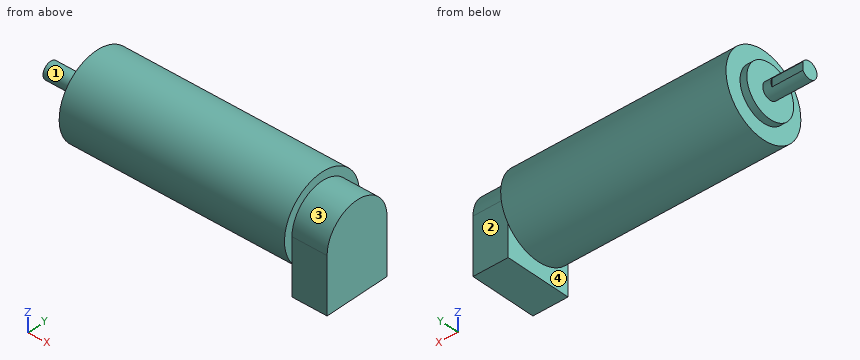
from build123d import *

# Parameters (mm, degrees)
SKETCH_2_R          = 20
EXTRUDE_1_DEPTH     = 109
EXTRUDE_2_DEPTH     = 17
SKETCH_5_R          = 12.5
EXTRUDE_3_DEPTH     = 3.3
SKETCH_6_R          = 4
EXTRUDE_4_DEPTH     = 19
CUT_EXTRUDE_START   = -15
CUT_EXTRUDE_1_DEPTH = 15


with BuildPart() as part:
    # 草图2 → 凸台-拉伸1 (new body)
    with BuildSketch(Plane(origin=(0, 0, 0), x_dir=(0, 0, -1), z_dir=(1, 0, 0))):
        Circle(SKETCH_2_R)
    extrude(amount=EXTRUDE_1_DEPTH)

    # 草图4 → 凸台-拉伸2 (add)
    with BuildSketch(Plane(origin=(109, 0, 0), x_dir=(0, 0, -1), z_dir=(1, 0, 0))):
        with BuildLine():
            Line((0, 16), (27, 16))
            Line((27, 16), (27, -16))
            Line((27, -16), (0, -16))
            ThreePointArc((0, -16), (-16, 0), (0, 16))
        make_face()
    extrude(amount=EXTRUDE_2_DEPTH)

    # 草图5 → 凸台-拉伸3 (add)
    with BuildSketch(Plane.ZY):
        with Locations(Location((0, 0, 0), (0, 0, 180))):
            Circle(SKETCH_5_R)
    extrude(amount=EXTRUDE_3_DEPTH)

    # 草图6 → 凸台-拉伸4 (add)
    with BuildSketch(Plane.ZY.offset(3.3)):
        with Locations(Location((0, 0, 0), (0, 0, 180))):
            Circle(SKETCH_6_R)
    extrude(amount=EXTRUDE_4_DEPTH)

    # 草图7 → 切除-拉伸1 (cut)
    with BuildSketch(Plane.ZY.offset(22.3).offset(CUT_EXTRUDE_START)):
        with BuildLine():
            Line((-1.936491673, 3.5), (1.936491673, 3.5))
            ThreePointArc((1.936491673, 3.5), (0, 4), (-1.936491673, 3.5))
        make_face()
    extrude(amount=CUT_EXTRUDE_1_DEPTH, mode=Mode.SUBTRACT)


solid = part.part
Source: CAD feature listing. Evaluate the final solid. Frame: model axes, mm. Face numbers are marked on the shaded views. A direction names the side the tool comes from. Round coordinates to 2 decimals unless told otherwise and drop trailing zeros. Loops run counter-clockwise (first coordinate to the right, second up) from the corner with the lowest first, then second, coordinate; pieces in that order, holes last. Notation, with made-up numbers: (89.25, -29) -> (102.25, -29) arc R28 ccw to (102.25, -11) -> close; hole circle Ø11 at (51.25, -22.5). An arc over 180 degrees is marked (long way). Answer as a JSON object with one key per item and string values. Group by question number.
Q1. Access query for the marked faces 1, 2, 3 and 4. Directions: +Z, -Z, +X, -X, +Y, -Y. A direction counts if a zero-diameter tool reaches every point of the face in a straight line with its end or side. Return the directions, or none.
Q2. Ray query, line 1 (X direction, y = 5.5, z = -7.5); line 2 (Z direction, x = 4.5, y = -1); line 3 (X direction, y = -7, z = 10.5). Return the intervals inside material, ascending. Write a range as from..to.
Q3. Section query B-B (x = 34.5). Output: boundary loops of the cut face in (y, z).
Q4. Section query D-D (y = -8.5). Output: boundary loops of the cut face in (x, z), plus the area to 3 significant figures.
Q5. Section query A-A (y = 0). Output: boundary loops of the cut face in (x, z).
Q6. Section query C-C (z = -23). Output: boundary loops of the cut face in (x, y).
Q7. Contact query for flat-ended pins moving along their axis: P1, Ø1.2, axis at x = -11.5, z = -1, coming from the +Y side; P2, Ø3, axis at x = 39.5, y = 12.5, coming from the +Z side; P3, Ø3, axis at y = -4, z = -17.5, coming from the -X side. Output: stop coordinate, or through.
Completed:
{
 "1": {"face 1": "-X", "face 2": "+Z, -Z, +X, +Y", "face 3": "+Z, +X", "face 4": "-Z, -X"},
 "2": {"line 1": "-3.3..126", "line 2": "-19.97..19.97", "line 3": "0..126"},
 "3": {"outline": "circle Ø40 at (0, 0)"},
 "4": {"outline": "(-3.3, -9.17) -> (0, -9.17) -> (0, -18.1) -> (109, -18.1) -> (109, -27) -> (126, -27) -> (126, 13.56) -> (109, 13.56) -> (109, 18.1) -> (0, 18.1) -> (0, 9.17) -> (-3.3, 9.17) -> close", "area": "4,700 mm²"},
 "5": {"outline": "(-22.3, -4) -> (-3.3, -4) -> (-3.3, -12.5) -> (0, -12.5) -> (0, -20) -> (109, -20) -> (109, -27) -> (126, -27) -> (126, 16) -> (109, 16) -> (109, 20) -> (0, 20) -> (0, 12.5) -> (-3.3, 12.5) -> (-3.3, 4) -> (-22.3, 4) -> close"},
 "6": {"outline": "(109, -16) -> (126, -16) -> (126, 16) -> (109, 16) -> close"},
 "7": {"P1": "y = 3.5", "P2": "z = 16.7", "P3": "x = 0"}
}
